Can you work these out from the model? Positions are in its coordinate system, mm. Give positions to 0.01 mm unless a question says otherwise; leave off trailing zeros. Write each loop counter-clockwise with the first axis right and the second up, starting at its lowest first coordinate (ties: lowest second). Pieces come first, ordered by that corner, then holes.
1. Suppose I cut it at A-A (z = -82.55). Please give me the cut outline in (x, y).
2. If I drill on probe 1 along Z at (x, y) = (12, -1); probe 2 along Z at (x, y) = (7.25, -25.5); probe 3 along Y at (x, z) = (5, 15) (3 decimals), over which ranges is the centre line in solid material (lowest first)?
3. Suppose I cut it at B-B (x = 9.5). Give the number of separate pieces and of enclosed holes in the cut face, and give its area (3 significant figures).
4. I'm going to push flat-ended pins straight in: pin 1 (4 mm diameter, centred on x = 3.5, y = 27, fed in from -Z); pin 2 (4.5 mm diameter, centred on y = 14.55, z = -92.76, fed in from -X); pin 3 (5 mm diameter, centred on x = 4.5, y = -10.5, fed in from -Z); pin 4 (3 mm diameter, centred on y = 40.5, z = -36, fed in from +X). Where does each tip first touch, or does it pass through?
5. Suppose I cut it at C-C (y = -33). Please give me the cut outline in (x, z), and give its area (3 significant figures).
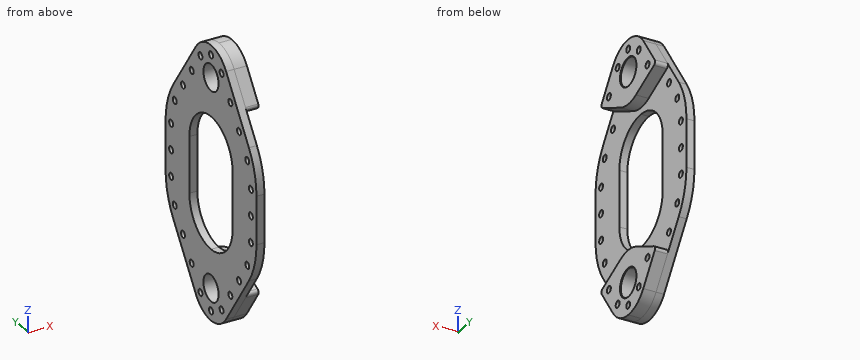
```python
from build123d import *
from build123d.topology import SkipClean

# Parameters (mm, degrees)
BOSS_EXTRUDE1_DEPTH    = 6.35
CUT_EXTRUDE3_START     = -6.35
CUT_EXTRUDE3_OUTLINE_R = 2.69253261
CUT_EXTRUDE3_DEPTH     = 6.35
SKETCH5_W              = 104.14
SKETCH5_H              = 59.69
CUT_EXTRUDE4_DEPTH     = 6.35
FILLET1_R              = 29.845
FILLET2_R              = 29.845
SKETCH14_R             = 2.69253261
BOSS_EXTRUDE3_DEPTH    = 10.16
FILLET3_R              = 2.54
FILLET3_OF_MIRROR1_R   = 2.54


# Read off the part's stored shape, not the designer's step: Cut-Extrude3
# Some blends are built 0.0001 mm under size
with BuildPart() as part:
    # Sketch1 → Boss-Extrude1 (new body)
    with BuildSketch(Plane(origin=(0, 0, 0), x_dir=(0, 0, -1), z_dir=(1, 0, 0))):
        with BuildLine():
            Line((19.05, 62.611), (-19.05, 62.611))
            ThreePointArc((-19.05, 62.611), (-36.688219036, 59.891543079), (-52.688239169, 51.985749479))
            Line((-52.688239169, 51.985749479), (-97.140382944, 20.791361801))
            ThreePointArc((-97.140382944, 20.791361801), (-107.949982522, -0.029797308), (-97.091561196, -20.82553716))
            Line((-97.091561196, -20.82553716), (-52.170359894, -52.19204611))
            ThreePointArc((-52.170359894, -52.19204611), (-36.41024798, -59.944824567), (-19.05, -62.611))
            Line((-19.05, -62.611), (19.05, -62.611))
            ThreePointArc((19.05, -62.611), (36.41024798, -59.944824567), (52.170359894, -52.19204611))
            Line((52.170359894, -52.19204611), (97.091561196, -20.82553716))
            ThreePointArc((97.091561196, -20.82553716), (107.949982522, -0.029797308), (97.140382944, 20.791361801))
            Line((97.140382944, 20.791361801), (52.688239169, 51.985749479))
            ThreePointArc((52.688239169, 51.985749479), (36.688219036, 59.891543079), (19.05, 62.611))
        make_face()
    extrude(amount=BOSS_EXTRUDE1_DEPTH)

    # Cut-Extrude3 outline → Cut-Extrude3 (cut)
    with BuildSketch(Plane(origin=(6.35, 0, 0), x_dir=(0, 0, -1), z_dir=(1, 0, 0)).offset(CUT_EXTRUDE3_START)):
        with Locations((0, 54.991)):
            Circle(CUT_EXTRUDE3_OUTLINE_R)
        with Locations((20.828, 54.959960993)):
            Circle(CUT_EXTRUDE3_OUTLINE_R)
        with Locations((41.055062572, 49.992917233)):
            Circle(CUT_EXTRUDE3_OUTLINE_R)
        with Locations((58.492960359, 38.603215535)):
            Circle(CUT_EXTRUDE3_OUTLINE_R)
        with Locations((75.541877036, 26.639101521)):
            Circle(CUT_EXTRUDE3_OUTLINE_R)
        with Locations((92.763268061, 14.553953261)):
            Circle(CUT_EXTRUDE3_OUTLINE_R)
        with Locations((100.329987765, -0.020858116)):
            Circle(CUT_EXTRUDE3_OUTLINE_R)
        with Locations((92.763268061, -14.553953261)):
            Circle(CUT_EXTRUDE3_OUTLINE_R)
        with Locations((-20.828, 54.959960993)):
            Circle(CUT_EXTRUDE3_OUTLINE_R)
        with Locations((-41.055062572, 49.992917233)):
            Circle(CUT_EXTRUDE3_OUTLINE_R)
        with Locations((-58.492960359, 38.603215535)):
            Circle(CUT_EXTRUDE3_OUTLINE_R)
        with Locations((-75.541877036, 26.639101521)):
            Circle(CUT_EXTRUDE3_OUTLINE_R)
        with Locations((-92.763268061, 14.553953261)):
            Circle(CUT_EXTRUDE3_OUTLINE_R)
        with Locations((-100.329987765, -0.020858116)):
            Circle(CUT_EXTRUDE3_OUTLINE_R)
        with Locations((-92.763268061, -14.553953261)):
            Circle(CUT_EXTRUDE3_OUTLINE_R)
        with Locations((-75.541877036, -26.639101521)):
            Circle(CUT_EXTRUDE3_OUTLINE_R)
        with Locations((-58.492960359, -38.603215535)):
            Circle(CUT_EXTRUDE3_OUTLINE_R)
        with Locations((-41.055062572, -49.992917233)):
            Circle(CUT_EXTRUDE3_OUTLINE_R)
        with Locations((-20.828, -54.959960993)):
            Circle(CUT_EXTRUDE3_OUTLINE_R)
        with Locations((0, -54.991)):
            Circle(CUT_EXTRUDE3_OUTLINE_R)
        with Locations((20.828, -54.959960993)):
            Circle(CUT_EXTRUDE3_OUTLINE_R)
        with Locations((41.055062572, -49.992917233)):
            Circle(CUT_EXTRUDE3_OUTLINE_R)
        with Locations((58.492960359, -38.603215535)):
            Circle(CUT_EXTRUDE3_OUTLINE_R)
        with Locations((75.541877036, -26.639101521)):
            Circle(CUT_EXTRUDE3_OUTLINE_R)
    extrude(amount=CUT_EXTRUDE3_DEPTH, mode=Mode.SUBTRACT)

    # Sketch5 → Cut-Extrude4 (cut)
    with BuildSketch(Plane(origin=(6.35, 0, 0), x_dir=(0, 0, -1), z_dir=(1, 0, 0))):
        Rectangle(SKETCH5_W, SKETCH5_H)
    extrude(amount=-CUT_EXTRUDE4_DEPTH, mode=Mode.SUBTRACT)

    # Fillet1
    fillet1_edges = [part.edges().sort_by_distance(p)[0] for p in [
        (3.175, -29.845, 52.07),
        (3.175, 29.845, 52.07),
    ]]
    fillet(fillet1_edges, radius=FILLET1_R - 0.0001)  # a hair under: the kernel refuses the full size

    # Fillet2
    fillet2_edges = [part.edges().sort_by_distance(p)[0] for p in [
        (3.175, 29.845, -52.07),
        (3.175, -29.845, -52.07),
    ]]
    fillet(fillet2_edges, radius=FILLET2_R - 0.0001)  # a hair under: the kernel refuses the full size

    # Sketch14 → Boss-Extrude3 (add)
    # profile 1 of 3: a face of its own
    with SkipClean():  # the faces are left unmerged after this step: merging them gives an invalid solid
        with BuildSketch(Plane(origin=(6.35, 0, 0), x_dir=(0, 0, -1), z_dir=(1, 0, 0))):
            with BuildLine():
                ThreePointArc((77.610004669, -24.914984369), (87.76808503, -24.858229797), (97.091561196, -20.82553716))
                ThreePointArc((97.091561196, -20.82553716), (105.072385024, -11.743175585), (107.95, 0))
                ThreePointArc((107.95, 0), (105.086145708, 11.716745991), (97.140382944, 20.791361801))
                ThreePointArc((97.140382944, 20.791361801), (87.797243185, 24.852091239), (77.610004669, 24.914984369))
                ThreePointArc((77.610004669, 24.914984369), (76.226910447, 24.03516967), (74.589917057, 24.120470135))
                ThreePointArc((74.589917057, 24.120470135), (65.621214015, 18.936108499), (59.468427534, 10.601934374))
                ThreePointArc((59.468427534, 10.601934374), (57.150017478, 0.029797308), (59.443616349, -10.547750213))
                ThreePointArc((59.443616349, -10.547750213), (65.599011292, -18.916235931), (74.589917057, -24.120470135))
                ThreePointArc((74.589917057, -24.120470135), (76.226910447, -24.03516967), (77.610004669, -24.914984369))
            make_face()
            with Locations((92.763268061, -14.553953261)):
                Circle(SKETCH14_R, mode=Mode.SUBTRACT)
            with Locations((100.329987765, -0.020858116)):
                Circle(SKETCH14_R, mode=Mode.SUBTRACT)
            with Locations((92.763268061, 14.553953261)):
                Circle(SKETCH14_R, mode=Mode.SUBTRACT)
        # profile 2 of 3: a face of its own
        with BuildSketch(Plane(origin=(6.35, 0, 0), x_dir=(0, 0, -1), z_dir=(1, 0, 0))):
            with BuildLine():
                ThreePointArc((77.610004669, 24.914984369), (87.797243185, 24.852091239), (97.140382944, 20.791361801))
                Line((97.140382944, 20.791361801), (72.190748783, 38.299821334))
                Line((72.190748783, 38.299821334), (59.468427534, 10.601934374))
                ThreePointArc((59.468427534, 10.601934374), (65.621214015, 18.936108499), (74.589917057, 24.120470135))
                ThreePointArc((74.589917057, 24.120470135), (74.011101322, 28.854154019), (78.234409646, 26.639101521))
                ThreePointArc((78.234409646, 26.639101521), (78.073500324, 25.722250725), (77.610004669, 24.914984369))
            make_face()
        # profile 3 of 3: a face of its own
        with BuildSketch(Plane(origin=(6.35, 0, 0), x_dir=(0, 0, -1), z_dir=(1, 0, 0))):
            with BuildLine():
                Line((72.100916604, -38.275410595), (97.091561196, -20.82553716))
                ThreePointArc((97.091561196, -20.82553716), (87.76808503, -24.858229797), (77.610004669, -24.914984369))
                ThreePointArc((77.610004669, -24.914984369), (78.073500324, -25.722250725), (78.234409646, -26.639101521))
                ThreePointArc((78.234409646, -26.639101521), (74.011101322, -28.854154019), (74.589917057, -24.120470135))
                ThreePointArc((74.589917057, -24.120470135), (65.599011292, -18.916235931), (59.443616349, -10.547750213))
                Line((59.443616349, -10.547750213), (72.100916604, -38.275410595))
            make_face()
        boss_extrude3 = extrude(amount=BOSS_EXTRUDE3_DEPTH)

    # Fillet3
    # the kernel refuses this fillet: 2.54 mm, written as the material it takes off along each edge
    with BuildSketch(Plane(origin=(6.35, -38.275410595, -72.100916604), x_dir=(0, 0.5725024092761827, -0.8199030377873753), z_dir=(1, 0, 0))) as fillet3_piece_1:
        with BuildLine():
            CenterArc((FILLET3_R * 1.2, FILLET3_R), FILLET3_R, 169.611142185, 100.388857815)
            Line((FILLET3_R * 0.216393442623, FILLET3_R * 1.18032786885), (0, 0))
            Line((0, 0), (FILLET3_R * 1.2, 0))
        make_face()
    extrude(amount=17.78, mode=Mode.SUBTRACT)
    with BuildSketch(Plane(origin=(6.35, 38.299821334, -72.190748783), x_dir=(0, -0.5744245253621356, -0.8185575512219561), z_dir=(1, 0, 0))) as fillet3_piece_2:
        with BuildLine():
            CenterArc((FILLET3_R * 1.2, -FILLET3_R), FILLET3_R, 90, 100.388857815)
            Line((FILLET3_R * 0.216393442623, -FILLET3_R * 1.18032786885), (0, 0))
            Line((0, 0), (FILLET3_R * 1.2, 0))
        make_face()
    extrude(amount=17.78, mode=Mode.SUBTRACT)

    # Sketch16 → 1/2 NPT Tapped Hole4 (revolve, cut)
    with SkipClean():  # the faces are left unmerged after this step: merging them gives an invalid solid
        with BuildSketch(Plane(origin=(16.51, 0, -82.55), x_dir=(0, 0, -1), z_dir=(0, 1, 0))):
            Polygon((0, 0), (0, 16.511), (8.9281, 16.511), (8.9281, 21.082), (10.273935163, 21.082), (10.8928789, 0.4101211), (11.303, 0), align=None)
        f_1_2_npt_tapped_hole4 = revolve(axis=Axis((22.86, 0, -82.55), (-1, 0, 0)), mode=Mode.SUBTRACT)

    # Mirror1: Boss-Extrude3, 1/2 NPT Tapped Hole4 across plane
    with SkipClean():  # the faces are left unmerged after this step: merging them gives an invalid solid
        add(boss_extrude3.mirror(Plane.XY))
        add(f_1_2_npt_tapped_hole4.mirror(Plane.XY), mode=Mode.SUBTRACT)

    # Fillet3 of Mirror1
    # the kernel refuses this fillet: 2.54 mm, written as the material it takes off along each edge
    with BuildSketch(Plane(origin=(6.35, -38.275410595, 72.100916604), x_dir=(0, 0.5725024092761827, 0.8199030377873753), z_dir=(1, 0, 0))) as fillet3_of_mirror1_piece_1:
        with BuildLine():
            CenterArc((FILLET3_OF_MIRROR1_R * 1.2, -FILLET3_OF_MIRROR1_R), FILLET3_OF_MIRROR1_R, 90, 100.388857815)
            Line((FILLET3_OF_MIRROR1_R * 0.216393442623, -FILLET3_OF_MIRROR1_R * 1.18032786885), (0, 0))
            Line((0, 0), (FILLET3_OF_MIRROR1_R * 1.2, 0))
        make_face()
    extrude(amount=17.78, mode=Mode.SUBTRACT)
    with BuildSketch(Plane(origin=(6.35, 38.299821334, 72.190748783), x_dir=(0, -0.5744245253621356, 0.8185575512219561), z_dir=(1, 0, 0))) as fillet3_of_mirror1_piece_2:
        with BuildLine():
            CenterArc((FILLET3_OF_MIRROR1_R * 1.2, FILLET3_OF_MIRROR1_R), FILLET3_OF_MIRROR1_R, 169.611142185, 100.388857815)
            Line((FILLET3_OF_MIRROR1_R * 0.216393442623, FILLET3_OF_MIRROR1_R * 1.18032786885), (0, 0))
            Line((0, 0), (FILLET3_OF_MIRROR1_R * 1.2, 0))
        make_face()
    extrude(amount=17.78, mode=Mode.SUBTRACT)


solid = part.part
```
Checks:
1. outline: (0, -30.98) - (16.51, -30.98) - (16.51, -11.3) - (16.1, -10.89) - (0, -10.41) - close; (0, 10.41) - (16.1, 10.89) - (16.51, 11.3) - (16.51, 31.03) - (0, 31.03) - close
2. probe 1: z = -107.93 to -102.84, -97.82 to -93.27, -71.83 to -57.17, 57.17 to 71.83, 93.27 to 97.82, 102.84 to 107.93
2. probe 2: z = -90.4 to -77.98, -73.1 to -66.27, 66.27 to 73.1, 77.98 to 90.4
2. probe 3: y = -62.611 to -29.845, 29.845 to 62.611
3. separate pieces: 2
3. enclosed holes: 12
3. area: 3,930 mm2
4. pin 1: stops at z = -91.14
4. pin 2: passes through
4. pin 3: stops at z = -106.66
4. pin 4: stops at x = 6.35
5. outline: (0, -79.66) - (16.51, -79.66) - (16.51, -69.69) - (6.35, -69.69) - (6.35, 69.69) - (16.51, 69.69) - (16.51, 79.66) - (0, 79.66) - close
5. area: 1,210 mm2
